The listing builds one solid part. Answer for the finished solid, in the listing's coordinates (mm). A direction names the side the tool comes from. Coordinates: 2 decimals unless noted, no trailing zeros. Order: outer loops, then holes, each group sorted by start corner. A loop starts at its lowest first (then second) coordinate and runs counter-clockwise, first axis right, second up. Notation, with made-up numbers: (38, 20.5) -> (96, 20.5) arc R19 cw to (96, 25.5) -> close; hole circle Ø2 at (8, 1.5). An arc over 180 degrees is marked (long way). Put each result on its own line as item: value. Start each with the question number.
```python
from build123d import *

# Parameters (mm, degrees)
SKETCH_1_W          = 30
SKETCH_1_H          = 60
EXTRUDE_1_DEPTH     = 12.5
SKETCH_2_R          = 9
EXTRUDE_2_DEPTH     = 4
SKETCH_3_R          = 6.25
EXTRUDE_3_DEPTH     = 2
FILLET_1_R          = 2
CUT_EXTRUDE_1_DEPTH = 10


with BuildPart() as part:
    # 草图1 → 凸台-拉伸1 (new body)
    with BuildSketch(Plane.XY):
        Rectangle(SKETCH_1_W, SKETCH_1_H)
    extrude(amount=EXTRUDE_1_DEPTH)

    # 草图2 → 凸台-拉伸2 (add)
    with BuildSketch(Plane.XY.offset(12.5)):
        with Locations(Location((0, 17, 0), (0, 0, 180))):
            Circle(SKETCH_2_R)
        with Locations(Location((0, -17, 0), (0, 0, 180))):
            Circle(SKETCH_2_R)
    extrude(amount=EXTRUDE_2_DEPTH)

    # 草图3 → 凸台-拉伸3 (add)
    with BuildSketch(Plane.XY.offset(16.5)):
        with Locations((0, 17)):
            Circle(SKETCH_3_R)
        with Locations((0, -17)):
            Circle(SKETCH_3_R)
    extrude(amount=EXTRUDE_3_DEPTH)

    # 圆角1
    fillet_1_edges = [part.edges().sort_by_distance(p)[0] for p in [
        (15, -30, 6.25),
        (-15, -30, 6.25),
        (-15, 30, 6.25),
        (15, 30, 6.25),
    ]]
    fillet(fillet_1_edges, radius=FILLET_1_R)

    # 草图4 → 切除-拉伸1 (cut)
    with BuildSketch(Plane.ZY.offset(15)):
        with BuildLine():
            ThreePointArc((10.25, 0), (8.751434736, 3.12134975), (5.37858787, 3.903926344))
            Line((5.37858787, 3.903926344), (6.25, 0))
            Line((6.25, 0), (10.25, 0))
        make_face()
        with BuildLine():
            Line((6.25, 0), (5.37858787, 3.903926344))
            ThreePointArc((5.37858787, 3.903926344), (3.12865025, 2.501434736), (2.25, 0))
            Line((2.25, 0), (6.25, 0))
        make_face()
        with BuildLine():
            Line((10.25, 0), (6.25, 0))
            Line((6.25, 0), (7.12141213, -3.903926344))
            ThreePointArc((7.12141213, -3.903926344), (9.37134975, -2.501434736), (10.25, 0))
        make_face()
        with BuildLine():
            Line((7.12141213, -3.903926344), (6.25, 0))
            Line((6.25, 0), (2.25, 0))
            ThreePointArc((2.25, 0), (3.748565264, -3.12134975), (7.12141213, -3.903926344))
        make_face()
    extrude(amount=-CUT_EXTRUDE_1_DEPTH, mode=Mode.SUBTRACT)


solid = part.part
```
(1) A tool of negligible diameter and unlimited length cuts with its end or side. For faces 4 (the flat face through (-5, 0, 6)), 5 (the cylindrical face through (7.14, 22.48, 14.47)), 6 (the cylindrical face through (14.4, 29.43, 6.34)), from which of +Z, -Z, +X, -X, +Y, -Y can it reach the whole face along a straight path? Write none if from no direction.
(2) For a pull along Y with two mould halves and no side action, classify faces 1 (the flat face through (0, -30, 6)), 2 (the cylindrical face through (-14.43, 29.4, 6.34)), 3 (the cylindrical face through (-1.355, 10.899, 17.486)) as released by +Y, released by -Y, zero draft, split by the parting line, or undercut.
(3) The part is cut by section B-B on y = 17. Determine the outline of the cut face in (x, z), plus the area to 3 significant figures.
(4) Find the intervals of material crossed by L1, parallel to X at y = 1, z = 5.5; L2, parallel to Z at x = 6, y = 22; L3, parallel to Z at x = 0.5, y = -0.5, in increasing order.
(5) The part is cut by section D-D on z = 8. Determine the outline of the cut face in (x, y).
(6) Each of these flat-tipped pins is pushed along its axis until it touches: P1, Ø6, axis at x = 1, y = 7.5, coming from the -Z side; P2, Ø5, axis at x = -10.5, y = 11, coming from the +Z side. Where does it stop, or does it pass through?
(7) The part is cut by section C-C on x = 0. Determine the outline of the cut face in (y, z), plus the area to 3 significant figures.
(8) The part is cut by section A-A on x = -12.25. Determine the outline of the cut face in (y, z), plus the area to 3 significant figures.
Worked out:
1. face 4: -X
1. face 5: +Z
1. face 6: +Z, -Z, +X, +Y
2. face 1: released by -Y
2. face 2: released by +Y
2. face 3: undercut
3. outline: (-15, 0) -> (15, 0) -> (15, 12.5) -> (9, 12.5) -> (9, 16.5) -> (6.25, 16.5) -> (6.25, 18.5) -> (-6.25, 18.5) -> (-6.25, 16.5) -> (-9, 16.5) -> (-9, 12.5) -> (-15, 12.5) -> close
3. area: 472 mm2
4. L1: -5 to 15
4. L2: 0 to 16.5
4. L3: 0 to 12.5
5. outline: (-15, -28) arc R2 ccw to (-13, -30) -> (13, -30) arc R2 ccw to (15, -28) -> (15, 28) arc R2 ccw to (13, 30) -> (-13, 30) arc R2 ccw to (-15, 28) -> (-15, 3.6) -> (-5, 3.6) -> (-5, -3.6) -> (-15, -3.6) -> close
6. P1: z = 0
6. P2: z = 12.5
7. outline: (-30, 0) -> (30, 0) -> (30, 12.5) -> (26, 12.5) -> (26, 16.5) -> (23.25, 16.5) -> (23.25, 18.5) -> (10.75, 18.5) -> (10.75, 16.5) -> (8, 16.5) -> (8, 12.5) -> (-8, 12.5) -> (-8, 16.5) -> (-10.75, 16.5) -> (-10.75, 18.5) -> (-23.25, 18.5) -> (-23.25, 16.5) -> (-26, 16.5) -> (-26, 12.5) -> (-30, 12.5) -> close
7. area: 944 mm2
8. outline: (-30, 0) -> (30, 0) -> (30, 12.5) -> (-30, 12.5) -> close; hole circle Ø8 at (0, 6.25)
8. area: 700 mm2
